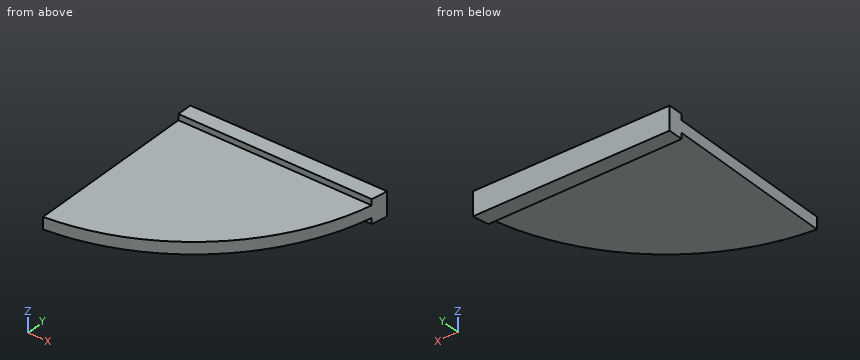
Autodesk Inventor part; units mm, degrees
ref_plane "YZ Plane" through (0, 0, 0) normal (1, 0, 0) x (0, 1, 0)
ref_plane "XZ Plane" through (0, 0, 0) normal (0, 1, 0) x (-1, 0, 0)
ref_plane "XY Plane" through (0, 0, 0) normal (0, 0, 1) x (1, 0, 0)
sketch "Sketch1" plane through (0, 0, 0) normal (0, 0, 1) x (1, 0, 0)
  line L0 (12.2331, 11.5545) -> (-8.7602, 11.5545)
  line L1 (-8.7602, 11.5545) -> (-8.7602, -8.5579)
  arc A0 (-8.7602, -8.5579) -> (12.2331, 11.5545) centre (-10.663, 14.4408) ccw
  point P0 (0, 0)
extrude "Extrusion1" add sketch "Sketch1" along normal mid plane 2.54
sketch "Sketch2" plane through (0, 0, 1.27) normal (0, 0, 1) x (1, 0, 0)
  line L0 (-8.7602, 11.5545) -> (-8.7602, -8.5579)
  line L1 (-8.7602, 9.9328) -> (11.9484, 9.8273)
  arc A0 (-8.7602, -8.5579) -> (12.2331, 11.5545) centre (-10.663, 14.4408) ccw
  point P0 (0, 0)
extrude "Extrusion2" cut sketch "Sketch2" against normal blind 0.635
sketch "Sketch3" plane through (0, 0, -1.27) normal (0, 0, -1) x (-1, 0, 0)
  line L0 (8.7602, 9.9328) -> (-11.9484, 9.8273)
  line L1 (8.7602, -8.5579) -> (8.7602, 11.5545)
  line L2 (8.7602, 9.9328) -> (8.7602, -8.5579)
  arc A0 (-11.9484, 9.8273) -> (8.7602, -8.5579) centre (10.663, 14.4408) ccw
  point P0 (0, 0)
extrude "Extrusion3" cut sketch "Sketch3" against normal blind 0.635
properties part number "Control surface"
Part model, mm, in its own coordinate system. Round coordinates to 2 decimals unless told otherwise and drop trailing zeros. Loops run counter-clockwise (first coordinate to the right, second up) from the corner with the lowest first, then second, coordinate; pieces in that order, holes last. Notation, with made-up numbers: (38, 3.25) -> (96, 3.25) arc R21 ccw to (96, 12.25) -> close; hole circle Ø4 at (36, 49.5). An arc over 180 degrees is marked (long way). Use one line per item in the form item = value. Start each with the question number.
Item 1: Drop flat-ended pins along their axis: pin 1 Ø2 at (x, y) = (10, 4.5) entering from +Z (3 decimals); pin 2 Ø1 at (x, y) = (-4, 6.5) entering from -Z (3 decimals); pin 3 Ø1 at (x, z) = (-2, -0.5) entering from -Y. Give the stop position or say it passes through.
Item 2: Drill centre lines: line 1 along Z through (x, y) = (-2.75, 0.25) (3 decimals); line 2 along Y through (x, z) = (10.75, 0.7); line 3 along Y through (x, z) = (-0.75, 0.7). Where is each one in solid material? Low to high.
Item 3: Band-saw the part on A-A (x = 1). List the corners of the cut face in (y, z) (1 decimal).
Item 4: Band-saw the part on D-D (x = 10). List the corners of the cut face in (y, z) (1 decimal), plus the area to 3 significant figures.
Item 5: Band-saw the part on B-B (z = 0.9). List the corners of the cut face in (x, y), plus the area to 3 significant figures.
Item 6: Band-saw the part on C-C (y = -1.75). List the corners of the cut face in (x, z) (3 decimals).
Data:
q1.pin_1 = 0.635
q1.pin_2 = -0.635
q1.pin_3 = -7.14
q2.line_1 = -0.635 to 0.635
q2.line_2 = 9.83 to 11.55
q2.line_3 = 9.89 to 11.55
q3.outline = (-5.5, -0.6) -> (9.9, -0.6) -> (9.9, -1.3) -> (11.6, -1.3) -> (11.6, 1.3) -> (9.9, 1.3) -> (9.9, 0.6) -> (-5.5, 0.6) -> close
q4.outline = (4.2, -0.6) -> (9.8, -0.6) -> (9.8, -1.3) -> (11.6, -1.3) -> (11.6, 1.3) -> (9.8, 1.3) -> (9.8, 0.6) -> (4.2, 0.6) -> close
q4.area = 11.6 mm^2
q5.outline = (-8.76, 9.93) -> (11.95, 9.83) arc R23.08 ccw to (12.23, 11.55) -> (-8.76, 11.55) -> close
q5.area = 34.9 mm^2
q6.outline = (-8.76, -0.635) -> (5.781, -0.635) -> (5.781, 0.635) -> (-8.76, 0.635) -> close
